Could you check a few things on this model? Use its own coordinates, in mm. A direction names the side the tool comes from. Coordinates: 2 decimals unless noted, no trailing zeros. Loops run counter-clockwise (first coordinate to the right, second up) from the corner with the lowest first, then second, coordinate; pieces in that order, holes last.
from build123d import *

# Parameters (mm, degrees)
EXTRUDE_1_DEPTH              = 0.5
SKETCH_2_R                   = 2.5
EXTRUDE_2_DEPTH              = 5
HOLE_WIZARD_M3_1_D           = 2.5
HOLE_WIZARD_M3_1_DEPTH       = 4
HOLE_WIZARD_M3_1_CSINK_D     = 3.05
HOLE_WIZARD_M3_1_CSINK_ANGLE = 90
HOLE_WIZARD_M3_1_TIP         = 0.751075774


with BuildPart() as part:
    # 草图1 → 凸台-拉伸1 (new body)
    with BuildSketch(Plane(origin=(0, 0, 0), x_dir=(1, 0, 0), z_dir=(0, 1, 0))):
        Polygon((0, -3.175426481), (2.75, -1.58771324), (2.75, 1.58771324), (0, 3.175426481), (-2.75, 1.58771324), (-2.75, -1.58771324), align=None)
    extrude(amount=EXTRUDE_1_DEPTH)

    # 草图2 → 凸台-拉伸2 (add)
    with BuildSketch(Plane(origin=(0, 0.5, 0), x_dir=(1, 0, 0), z_dir=(0, 1, 0))):
        Circle(SKETCH_2_R)
    extrude(amount=EXTRUDE_2_DEPTH)

    # M3 螺纹孔1
    with Locations(Plane(origin=(0, 5.5, 0), x_dir=(1, 0, 0), z_dir=(0, 1, 0))):
        with Locations((0, 0)):
            CounterSinkHole(HOLE_WIZARD_M3_1_D / 2, HOLE_WIZARD_M3_1_CSINK_D / 2, depth=HOLE_WIZARD_M3_1_DEPTH, counter_sink_angle=HOLE_WIZARD_M3_1_CSINK_ANGLE)
            with Locations((0, 0, -(HOLE_WIZARD_M3_1_DEPTH + HOLE_WIZARD_M3_1_TIP / 2))):  # 118° drill point
                Cone(0, HOLE_WIZARD_M3_1_D / 2, HOLE_WIZARD_M3_1_TIP, mode=Mode.SUBTRACT)


solid = part.part
1) Imagine slicing it at B-B on z = 1.75. List the corners of the cut face in (x, y) for me.
2) Imagine slicing it at C-C on x = 1.9. List the corners of the cut face in (y, z) for me, plus the area to 3 significant figures.
3) Imagine slicing it at A-A on y = 3.3. List the corners of the cut face in (x, z) for me, plus the area to 3 significant figures.
4) If I drill on L1, parallel to Z at x = 0, y = 2.6; L2, parallel to Y at x = -0.95, z = -2.5; L3, parallel to Z at x = 0.85, y = 2.9, over which ranges is the centre line in solid material (lowest first)?
5) Will these pins go through, and if not, where does the flat tip stop? pin 1 (2 mm diameter, centred on y = 2, z = 2, fed in from +X); pin 2 (2 mm diameter, centred on x = 0, z = 0, fed in from +Y); pin 3 (2 mm diameter, centred on x = 0, y = 3, fed in from -Z).
6) We'd pull the mould along X, two halves only. Please class faces 1 (the conical face through (-0.05, 0.88, 0.21)), 2 (the flat face through (0, 0, 0)), 3 (the flat face through (-1.394, 0.246, 2.37)), 4 (the cylindrical face through (0.27, 3.34, 1.22)): released by +X, released by -X, zero draft, split by the parting line, or undercut.
7) For faces 5 (the flat face through (0, 0.5, 3)), 6 (the flat face through (0, 5.5, 2)), which set-ups out of +Z, -Z, +X, -X, +Y, -Y let a thin tool reach every point of the face, with its end or its side?
Solved:
1. outline: (-2.47, 0) - (2.47, 0) - (2.47, 0.5) - (1.79, 0.5) - (1.79, 5.5) - (-1.79, 5.5) - (-1.79, 0.5) - (-2.47, 0.5) - close
2. outline: (0, -2.08) - (0.5, -2.08) - (0.5, -1.62) - (5.5, -1.62) - (5.5, 1.62) - (0.5, 1.62) - (0.5, 2.08) - (0, 2.08) - close
2. area: 18.3 mm2
3. outline: circle Ø5 at (0, 0); hole circle Ø2.5 at (0, 0)
3. area: 14.7 mm2
4. L1: z = -2.5 to -1.25, 1.25 to 2.5
4. L2: y = 0 to 0.5
4. L3: z = -2.35 to -0.92, 0.92 to 2.35
5. pin 1: stops at x = 2.29
5. pin 2: stops at y = 1.35
5. pin 3: stops at z = -2.5
6. face 1: undercut
6. face 2: zero draft
6. face 3: released by -X
6. face 4: undercut
7. face 5: +Y
7. face 6: +Z, -Z, +X, -X, +Y
